Read the model definition and answer for the solid it produces. Units are mm, in the model's axes. Give positions to 0.01 mm unless a question says otherwise; leave off trailing zeros. Order: outer loops, then holes, each group sorted by start corner. A loop starts at its lowest first (then second) coordinate and runs counter-clockwise, first axis right, second up. Notation, with made-up numbers: (1.25, -3.5) -> (42.25, -3.5) arc R10 cw to (42.25, 8.5) -> close; hole circle Ø9 at (54.5, -27.75). An arc over 180 degrees is marked (long way). One line per item, written item: value. Start each with the question number.
from build123d import *

# Parameters (mm, degrees)
SKETCH1_W                  = 200
SKETCH1_H                  = 160
BASE_DEPTH                 = 20
SKETCH2_R                  = 30
ACTUATOR_CUT_DEPTH         = 40
F_12_0MM_DOWEL_HOLE1_D     = 12
F_12_0MM_DOWEL_HOLE1_DEPTH = 20


with BuildPart() as part:
    # Sketch1 → base (new body)
    with BuildSketch(Plane(origin=(0, 0, 0), x_dir=(1, 0, 0), z_dir=(0, 1, 0))):
        Rectangle(SKETCH1_W, SKETCH1_H)
    extrude(amount=BASE_DEPTH)

    # Sketch2 → actuator cut (cut)
    with BuildSketch(Plane(origin=(0, 20, 0), x_dir=(1, 0, 0), z_dir=(0, 1, 0))):
        Circle(SKETCH2_R)
    extrude(amount=-ACTUATOR_CUT_DEPTH, mode=Mode.SUBTRACT)

    # Ø12.0mm Dowel Hole1
    with Locations(Plane(origin=(55, 20, -55), x_dir=(0, 0, 1), z_dir=(0, 1, 0))):
        with Locations((0, 0), (0, -110), (110, -110), (110, 0)):
            Hole(F_12_0MM_DOWEL_HOLE1_D / 2, depth=F_12_0MM_DOWEL_HOLE1_DEPTH)


solid = part.part
Item 1: A flat-ended cylindrical pin translates along its axis: pin 1 (7 mm diameter, centred on x = 55, z = 55, fed in from -Y). Find the tip coordinate at first contact, or state that the pin passes through.
Item 2: Find section C-C on z = 55. Write down the section's boundary in (x, y).
Item 3: For a pull along Z with two mould halves and no side action, classify faces 1 (the cylindrical face through (55, 10, 61)), 2 (the flat face through (-100, 10, 1)), 3 (the flat face through (-1, 10, 80)) as +Z half, -Z half, draft (parallel to the pull), parting line (faces both ways), or undercut.
Item 4: Find section D-D on x = 55. Write down the section's boundary in (y, z).
Item 5: Find section A-A on y = 7.25. Write down the section's boundary in (x, z).
Item 6: Find section B-B on x = 0. Write down the section's boundary in (y, z).
Item 7: Find the intervals of material crossed by line 1 (X direction, y = 7.75, z = -55); line 2 (X direction, y = 7, z = 0); line 3 (X direction, y = 2.5, z = 49.5), in increasing order. Write a range as from..to.
Checks:
1. pin 1: through
2. outline: (-100, 0) -> (-61, 0) -> (-61, 20) -> (-100, 20) -> close; (-49, 0) -> (49, 0) -> (49, 20) -> (-49, 20) -> close; (61, 0) -> (100, 0) -> (100, 20) -> (61, 20) -> close
3. face 1: undercut
3. face 2: draft
3. face 3: +Z half
4. outline: (0, -80) -> (20, -80) -> (20, -61) -> (0, -61) -> close; (0, -49) -> (20, -49) -> (20, 49) -> (0, 49) -> close; (0, 61) -> (20, 61) -> (20, 80) -> (0, 80) -> close
5. outline: (-100, -80) -> (100, -80) -> (100, 80) -> (-100, 80) -> close; hole circle Ø12 at (-55, -55); hole circle Ø12 at (-55, 55); hole circle Ø60 at (0, 0); hole circle Ø12 at (55, -55); hole circle Ø12 at (55, 55)
6. outline: (0, -80) -> (20, -80) -> (20, -30) -> (0, -30) -> close; (0, 30) -> (20, 30) -> (20, 80) -> (0, 80) -> close
7. line 1: -100..-61, -49..49, 61..100
7. line 2: -100..-30, 30..100
7. line 3: -100..-57.4, -52.6..52.6, 57.4..100
